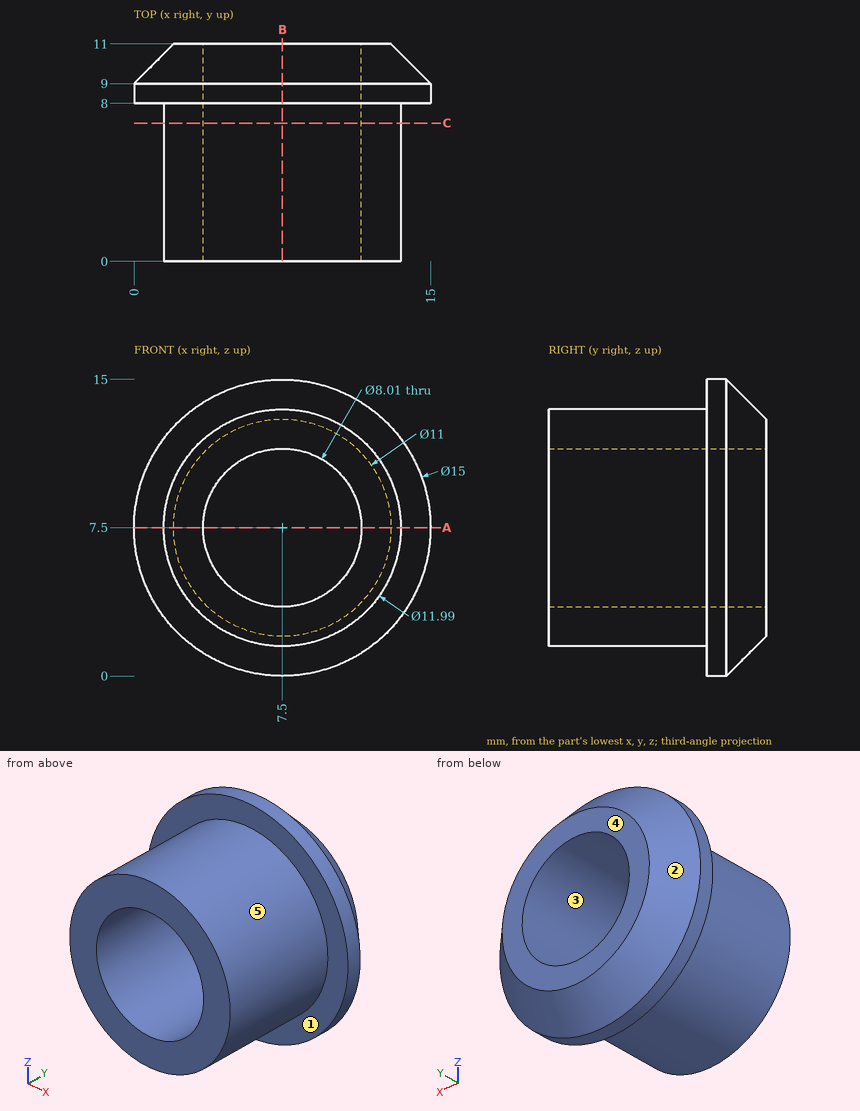
The figure shows three views and two pictorial views of one solid part (mm, origin at its lowest corner). Answer the questions. A direction names the side the tool comes from. Give positions to 0.01 mm unless a question says otherwise; leave off trailing zeros. Order: outer loops, then holes, each group sorted by start corner. A loop starts at its lowest first (then second) coordinate and runs counter-clockwise, first axis right, second up. Notation, with made-up numbers: (25, 35.5) -> (60, 35.5) arc R29 ccw to (60, 57.5) -> close; hole circle Ø5 at (21.25, -13.5). An arc over 180 degrees is marked (long way). One line per item, written item: value.
1) Find the intervals of material crossed by line 1 (X direction, y = 3, z = 7.5) (3 decimals); line 2 (Z direction, x = 6.25, y = 5.5); line 3 (Z direction, x = 8.5, y = 2.5), in increasing order.
Reported:
line 1: x = 1.505 to 3.495, 11.505 to 13.495
line 2: z = 1.64 to 3.7, 11.3 to 13.36
line 3: z = 1.59 to 3.62, 11.38 to 13.41
2) Determine the mould class of the marked faces 1, 2 and 3 for opening direction Z: pulls with the +Z half, pulls with the -Z half, needs draft (parallel to the pull), parting line crosses it, or undercut.
Reported:
face 1: needs draft
face 2: parting line crosses it
face 3: undercut
3) Find section A-A, the plane z = 7.5. Determine the outline of the cut face in (x, y) (3 decimals), plus the area to 3 significant figures.
Reported:
outline: (0, 8) -> (1.505, 8) -> (1.505, 0) -> (3.495, 0) -> (3.495, 11) -> (2, 11) -> (0, 9) -> close; (11.505, 0) -> (13.495, 0) -> (13.495, 8) -> (15, 8) -> (15, 9) -> (13, 11) -> (11.505, 11) -> close
area: 48.8 mm^2
4) A tool of negligible diameter and unlimited length cuts with its end or side. For the marked faces 4 and 5, from which of +Z, -Z, +X, -X, +Y, -Y can it reach the whole face along a straight path? Write none if from no direction.
Reported:
face 4: +Z, -Z, +X, -X, +Y
face 5: -Y
5) Find section B-B, the plane x = 7.5. Determine the outline of the cut face in (y, z) (3 decimals).
Reported:
outline: (0, 1.505) -> (8, 1.505) -> (8, 0) -> (9, 0) -> (11, 2) -> (11, 3.495) -> (0, 3.495) -> close; (0, 11.505) -> (11, 11.505) -> (11, 13) -> (9, 15) -> (8, 15) -> (8, 13.495) -> (0, 13.495) -> close
6) Find section C-C, the plane y = 7. Determine the outline of the cut face in (x, z) (3 decimals).
Reported:
outline: circle Ø11.99 at (7.5, 7.5); hole circle Ø8.01 at (7.5, 7.5)
7) Flat-ended cylindrical pins translate along their axes: P1, Ø3, axis at x = 10.5, y = 5.5, coming from the -Z side; P2, Ø1, axis at x = 13, y = 3, coming from the +Z side; P3, Ø3, axis at x = 11, y = 2, coming from the +Z side. Find the tip coordinate at first contact, or state that the pin passes through.
Reported:
P1: stops at z = 1.7
P2: stops at z = 10.81
P3: stops at z = 13.15
